Verification items for the finished model (mm, model axes). Face numbers are marked on the shaded views. Coordinates: 2 decimals unless noted, no trailing zeros. Write each loop counter-clockwise with the first axis right and the second up, starting at its lowest first coordinate (ties: lowest second). Pieces come first, ordered by that corner, then holes. Notation, with made-up numbers: (82.25, 89) -> (106.25, 89) arc R26 cw to (106.25, 123) -> close; hole circle Ø11 at (22, -32). An arc over 180 degrees is marked (long way). Write each question's results on one line, items separated by ' | '. Start each with the question number.
from build123d import *

# Parameters (mm, degrees)
CYLINDER1726_R              = 1.5
CYLINDER1726_DEPTH          = 50
COMPOUND868_PLACEMENT_ANGLE = 225
CYLINDER1725_R              = 1.5
CYLINDER1725_DEPTH          = 50
COMPOUND869_PLACEMENT_ANGLE = 225
CYLINDER1724_R              = 74
CYLINDER1724_DEPTH          = 40
BOX685_W                    = 42
BOX685_H                    = 8
BOX685_DEPTH                = 18
COMPOUND862_PLACEMENT_ANGLE = 225


with BuildPart() as compound868:
    # Cylinder1726 → Cylinder1726 (new body)
    with BuildSketch(Plane(origin=(18, 100, 72), x_dir=(1, 0, 0), z_dir=(0, -1, 0))):
        Circle(CYLINDER1726_R)
    extrude(amount=CYLINDER1726_DEPTH)


with BuildPart() as compound868_1:
    # Compound868 placement: moved
    add(compound868.part.rotate(Axis((0, 0, 0), (0, 0, 1)), COMPOUND868_PLACEMENT_ANGLE))


with BuildPart() as compound867:
    # Cylinder1725 → Cylinder1725 (new body)
    with BuildSketch(Plane(origin=(-18, 100, 72), x_dir=(1, 0, 0), z_dir=(0, -1, 0))):
        Circle(CYLINDER1725_R)
    extrude(amount=CYLINDER1725_DEPTH)


with BuildPart() as compound867_1:
    # Compound869 placement: moved
    add(compound867.part.rotate(Axis((0, 0, 0), (0, 0, 1)), COMPOUND869_PLACEMENT_ANGLE))

    # Compound867: union Compound868
    add(compound868_1.part)


with BuildPart() as compound867_2:
    # Compound867 placement: moved
    add(compound867_1.part.moved(Location((0, 0, 1))))


with BuildPart() as obj1:
    # Cylinder1724 → Cylinder1724 (new body)
    with BuildSketch(Plane.XY.offset(44)):
        Circle(CYLINDER1724_R)
    extrude(amount=CYLINDER1724_DEPTH)


with BuildPart() as cut499:
    # Box685 → Box685 (new body)
    with BuildSketch(Plane(origin=(-21, -23, 22), x_dir=(1, 0, 0), z_dir=(0, 0, 1))):
        with Locations((21, 4)):
            Rectangle(BOX685_W, BOX685_H)
    extrude(amount=BOX685_DEPTH)


with BuildPart() as cut499_1:
    # Compound862 placement: moved
    add(cut499.part.moved(Location((63.64, -63.64, 43))).rotate(Axis((63.64, -63.64, 43), (0, 0, 1)), COMPOUND862_PLACEMENT_ANGLE))

    # Cut498: cut obj1
    add(obj1.part, mode=Mode.SUBTRACT)

    # Cut499: cut Compound867
    add(compound867_2.part, mode=Mode.SUBTRACT)


solid = cut499_1.part
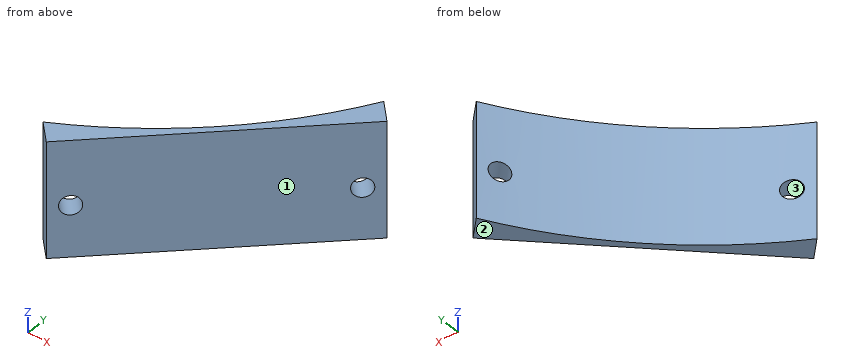
1. Sectioned sample at A-A on z = 74. Record the cut outline in (x, y), plus the area to 3 significant figures.
2. Depth check by flat-ended pin: pin 1 Ø6 at (y, z) = (-46, 79) entering from -X; pin 2 Ø12 at (x, y) = (46, -45.5) entering from -Z; pin 3 Ø10 at (x, z) = (58.5, 69) entering from -Y; pin 4 Ø5 at (y, z) = (-60, 68) entering from +X. Enter the tip coordinate at first touch or a pass-through.
3. Material ranges on probe 1 along Y at (x, z) = (50, 75.75); probe 2 along X at (y, z) = (-45.5, 74.75); probe 3 along Y at (x, z) = (53, 74), recorded low to high. Write a range as from..to.
4. Mould release check, pull along Y, two halves, no side actions. Record for the marked faces 1, 2 and 3: +Y half, -Y half, draft (parallel to the pull), parting line (faces both ways), or undercut.
5. Sectioned sample at B-B on z = 77.25. Record the cut outline in (x, y), plus the area to 3 significant figures.
6. Sectioned sample at C-C on x = 44. Record the cut outline in (y, z).
Computed values:
1) outline: (35.33, -65.02) -> (38.18, -67.88) -> (39.51, -66.55) -> (37.03, -64.07) arc R74 cw to start; (39.01, -62.88) -> (41.1, -64.97) -> (64.97, -41.1) -> (62.88, -39.01) arc R74 cw to start; (64.07, -37.03) -> (66.55, -39.51) -> (67.88, -38.18) -> (65.02, -35.33) arc R74 cw to start | area: 69.8 mm^2
2) pin 1: stops at x = 55.45 | pin 2: passes through | pin 3: stops at y = -52.57 | pin 4: stops at x = 48.57
3) probe 1: y = -56.07..-54.55 | probe 2: x = 58.36..60.57 | probe 3: y = -53.07..-51.64
4) face 1: -Y half | face 2: draft | face 3: undercut
5) outline: (35.33, -65.02) -> (38.18, -67.88) -> (67.88, -38.18) -> (65.02, -35.33) arc R74 cw to start | area: 84.3 mm^2
6) outline: (-62.07, 65) -> (-59.5, 65) -> (-59.5, 83) -> (-62.07, 83) -> close
